The listing builds one solid part. Answer for the finished solid, in the listing's coordinates (mm). A direction names the side the tool comes from. Give positions to 0.01 mm unless a question says otherwise; leave off trailing zeros. Write each loop counter-clockwise with the first axis right and the second up, starting at its lowest first coordinate (ties: lowest second). Pieces come first, ordered by that corner, then holes.
Autodesk Fusion 360 part; units mm, degrees
sketch "Switch" plane through (0, 0, 0) normal (0, 1, 0) x (1, 0, 0)
  line L0 (-7, 7) -> (7, 7)
  line L1 (-8.5, -8.5) -> (-8.5, 8.5)
  line L2 (7, -7) -> (-7, -7)
  line L3 (-8.5, 8.5) -> (8.5, 8.5)
  line L4 (-8.5, -8.5) -> (8.5, 8.5) construction
  line L5 (-7, -7) -> (7, 7) construction
  line L6 (8.5, -8.5) -> (-8.5, -8.5)
  line L7 (-7, -7) -> (-7, 7)
  line L8 (7, 7) -> (7, -7)
  line L9 (8.5, 8.5) -> (8.5, -8.5)
  line L10 (8.5, -8.5) -> (-8.5, 8.5) construction
  line L11 (7, -7) -> (-7, 7) construction
  line L12 (-12, 12) -> (12, 12)
  line L13 (12, 12) -> (12, -12)
  line L14 (12, -12) -> (-12, -12)
  line L15 (-12, -12) -> (-12, 12)
  line L16 (-12, 12) -> (12, -12) construction
  line L17 (12, 12) -> (-12, -12) construction
  dimension "d1" = 14
  dimension "d2" = 14
  dimension "d3" = 1.5
  dimension "d4" = 1.5
  dimension "d5" = 1.5
  dimension "d6" = 1.5
  dimension "d7" = 24
  dimension "d8" = 24
extrude "Switch Extrusion" add sketch "Switch" along normal blind 3 contours L12 L13 L14 L15
extrude "Switch Hole Extrusion" add sketch "Switch" along normal blind 1.3 contours L1 L3 L6 L9
Item 1: A cutting plane is placed at D-D, the plane x = 7.75. Give the vertices of the cut face in (y, z).
Conclusion:
outline: (0, -12) - (3, -12) - (3, -8.5) - (1.3, -8.5) - (1.3, 8.5) - (3, 8.5) - (3, 12) - (0, 12) - close
Item 2: A cutting plane is placed at B-B, the plane x = -1.5. Give the vertices of the cut face in (y, z), plus the area to 3 significant figures.
Conclusion:
outline: (0, -12) - (3, -12) - (3, -8.5) - (1.3, -8.5) - (1.3, -7) - (0, -7) - close; (0, 7) - (1.3, 7) - (1.3, 8.5) - (3, 8.5) - (3, 12) - (0, 12) - close
area: 24.9 mm2
Item 3: Consider probe 1 along Z at (x, y) = (-3, 2.1); probe 2 along X at (y, z) = (0.8, 5.25). Determine where each line is inside the solid, lowest interval first.
Conclusion:
probe 1: z = -12 to -8.5, 8.5 to 12
probe 2: x = -12 to -7, 7 to 12
Item 4: A cutting plane is placed at A-A, the plane z = -2. Give the vertices of the cut face in (x, y), plus the area to 3 significant figures.
Conclusion:
outline: (-12, 0) - (-7, 0) - (-7, 1.3) - (-8.5, 1.3) - (-8.5, 3) - (-12, 3) - close; (7, 0) - (12, 0) - (12, 3) - (8.5, 3) - (8.5, 1.3) - (7, 1.3) - close
area: 24.9 mm2
Item 5: Determine the mould class of faces 1 (the face through (0, 1, -12)), 2 (the face through (-8, 1.3, 0)), 3 (the face through (-8.5, 2, 0)), 4 (the face through (0, 1, 12)) for opening direction Z: pulls with the +Z half, pulls with the -Z half, needs draft (parallel to the pull), parting line crosses it, or undercut.
Conclusion:
face 1: pulls with the -Z half
face 2: undercut
face 3: undercut
face 4: pulls with the +Z half
Item 6: A cutting plane is placed at C-C, the plane y = 0.45. Give the vertices of the cut face in (x, z), plus the area to 3 significant figures.
Conclusion:
outline: (-12, -12) - (12, -12) - (12, 12) - (-12, 12) - close; hole (-7, -7) - (7, -7) - (7, 7) - (-7, 7) - close
area: 380 mm2
Item 7: Which of the six approach directions +Z, -Z, +X, -X, +Y, -Y give full straight-line access (tool end or side, diameter ignored) to faces 5 (the face through (0, 2, 8.5)), 6 (the face through (10, 3, 0)), 7 (the face through (-7, 1, 0))?
Conclusion:
face 5: +Y
face 6: +Z, -Z, +X, -X, +Y
face 7: +Y, -Y
Item 8: This flat-tipped pin is pushed along its axis until it touches: P1, Ø1.5, axis at x = 3.5, z = -6.5, coming from the +Y side. Where does it stop, or does it pass through?
Conclusion:
P1: stops at y = 1.3
